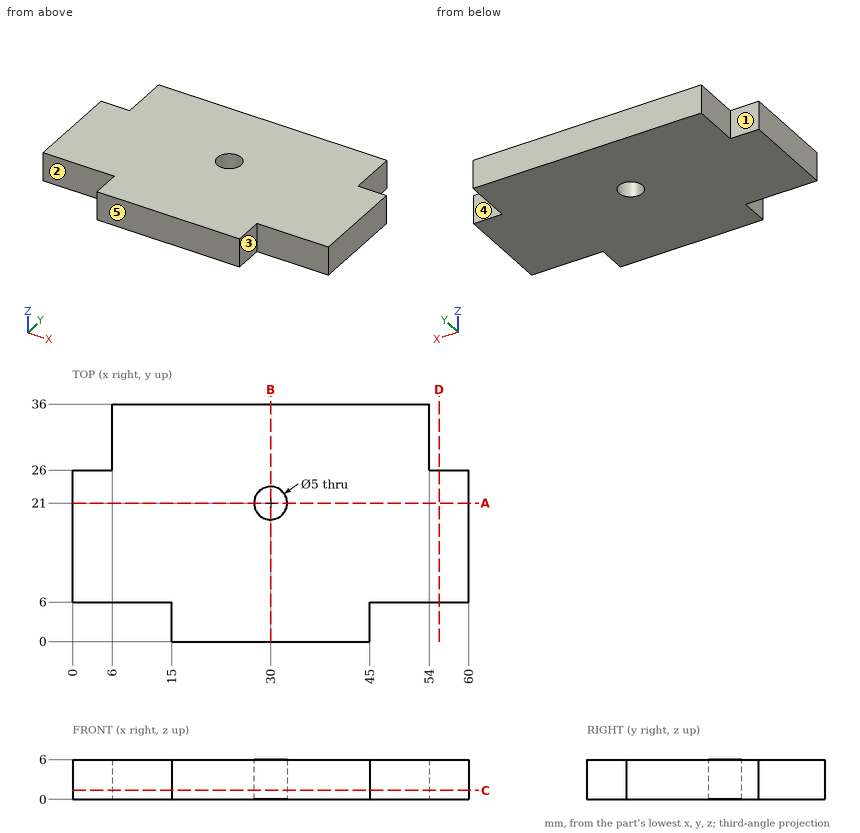
Print and shaded views of the part. All mm, measured from the part's lowest x, y and z. A direction names the side the tool comes from. Round coordinates to 2 decimals unless told otherwise and drop trailing zeros. Write each loop counter-clockwise with the first axis right and the second up, starting at its lowest first coordinate (ties: lowest second). Pieces come first, ordered by that corner, then holes. Notation, with made-up numbers: (81.5, 72.25) - (101.5, 72.25) arc R20 ccw to (101.5, 88.25) - close; hole circle Ø6 at (77, 39). An arc over 180 degrees is marked (long way). One line per item, written item: value.
(1) 3-axis set-ups, long thin cutter, end or side, ignore diameter. For the marked faces 1, 2, 3, 4 and 5: which of +Z, -Z, +X, -X, +Y, -Y reach the whole face in a straight line?
Values follow:
face 1: +Z, -Z, -X, +Y
face 2: +Z, -Z, -X, -Y
face 3: +Z, -Z, +X, -Y
face 4: +Z, -Z, +X, +Y
face 5: +Z, -Z, +X, -X, -Y
(2) Cut at C-C, the plane z = 1.35. Give the cut face in (x, y), plus the area to 3 significant figures.
Values follow:
outline: (0, 6) - (15, 6) - (15, 0) - (45, 0) - (45, 6) - (60, 6) - (60, 26) - (54, 26) - (54, 36) - (6, 36) - (6, 26) - (0, 26) - close; hole circle Ø5 at (30, 21)
area: 1,840 mm²
(3) Drop flat-ended pins along their axis: P1, Ø1.8, axis at x = 57, z = 2.5, coming from the +Y side; P2, Ø5, axis at x = 19.5, y = 16.5, coming from the -Z side; P3, Ø3, axis at y = 2.5, z = 4.5, coming from the +X side; P4, Ø1.8, axis at y = 29.5, z = 3, coming from the -X side. Give the stop position or say it passes through.
Values follow:
P1: stops at y = 26
P2: stops at z = 0
P3: stops at x = 45
P4: stops at x = 6
(4) Cut at D-D, the plane x = 55.5. Give the cut face in (y, z).
Values follow:
outline: (6, 0) - (26, 0) - (26, 6) - (6, 6) - close
(5) Cut at B-B, the plane x = 30. Give the cut face in (y, z).
Values follow:
outline: (0, 0) - (18.5, 0) - (18.5, 6) - (0, 6) - close; (23.5, 0) - (36, 0) - (36, 6) - (23.5, 6) - close
(6) Cut at A-A, the plane y = 21. Give the cut face in (x, z).
Values follow:
outline: (0, 0) - (27.5, 0) - (27.5, 6) - (0, 6) - close; (32.5, 0) - (60, 0) - (60, 6) - (32.5, 6) - close
(7) Wall check: probe 1 along Y at (x, z) = (30, 4.1); probe 2 along X at (y, z) = (4, 1.55); probe 3 along Y at (x, z) = (3, 0.6). Give the ranges that are in metal, low to high.
Values follow:
probe 1: y = 0 to 18.5, 23.5 to 36
probe 2: x = 15 to 45
probe 3: y = 6 to 26
